Here's how the part is built. I have some questions about the finished solid (model axes, mm). A direction names the side the tool comes from. Give positions to 0.01 mm unless a question says otherwise; leave off trailing zeros. Order: outer loops, then holes, each group sorted by start corner. A loop starts at its lowest first (then second) coordinate and runs counter-clockwise, first axis right, second up.
Autodesk Inventor part; units mm, degrees
ref_plane "YZ Plane" through (0, 0, 0) normal (1, 0, 0) x (0, 1, 0)
ref_plane "XZ Plane" through (0, 0, 0) normal (0, 1, 0) x (-1, 0, 0)
ref_plane "XY Plane" through (0, 0, 0) normal (0, 0, 1) x (1, 0, 0)
sketch "Sketch1" plane through (0, 0, 0) normal (1, 0, 0) x (0, 1, 0)
  line L0 (0, 0) -> (0, 8)
  line L1 (0, 8) -> (2.5, 8)
  circle A0 centre (2.5, 8) radius 1.05
  circle A1 centre (2.5, 8) radius 1.9
  dimension "d1" = 8
  dimension "d2" = 2.5
  dimension "d3" = 2.1
  dimension "d7" = 3.8
sketch "Sketch4" plane through (0, 0, 0) normal (1, 0, 0) x (0, 1, 0)
  line L0 (0, 0) -> (0, 3.5)
  line L1 (0, 3.5) -> (0, 12.5)
  line L2 (0, 12.5) -> (2.5, 12.5)
  line L3 (2.5, 12.5) -> (5.5, 12.5)
  line L4 (5.5, 12.5) -> (5.5, 9.5)
  line L5 (2.5, 12.5) -> (5.5, 9.5)
  line L6 (0, 0) -> (5.5, 0)
  line L7 (5.5, 0) -> (5.5, 9.5)
  dimension "d32" = 3.5
  dimension "d33" = 9
  dimension "d35" = 2.5
  dimension "d37" = 3
  dimension "d38" = 3
extrude "Extrusion3" add sketch "Sketch4" along normal blind 3 contours L0 L1 L2 L5 L7 L6
sketch "Sketch9" plane through (3, 0, 0) normal (1, 0, 0) x (0, 0, -1)
  line L0 (0, 0) -> (-3.5, 0)
  line L1 (-12.5, 0) -> (0, 0)
  line L2 (-3.5, 0) -> (-4.5, 0)
  line L3 (-3.5, 0) -> (-3.5, 2.5)
  line L4 (-3.5, 2.5) -> (-4.5, 2.5)
  line L5 (-4.5, 2.5) -> (-4.5, 0)
  line L6 (-4.5, 0) -> (-11.5, 0)
  line L7 (-11.5, 2.5) -> (-12.5, 2.5)
  line L8 (-11.5, 2.5) -> (-11.5, 0)
  line L9 (-12.5, 2.5) -> (-12.5, 0)
  line L10 (-12.5, 0) -> (-11.5, 0)
  dimension "d70" = 3.5
  dimension "d71" = 1
  dimension "d72" = 1
  dimension "d73" = 7
  dimension "d74" = 2.5
extrude "Extrusion4" add sketch "Sketch9" along normal blind 2 contours L9 L7 L8 L1
sketch "Sketch10" plane through (0, 0, 12.5) normal (0, 0, 1) x (1, 0, 0)
  line L0 (3, 0) -> (3, 5.5)
  line L1 (3, 0) -> (5, 0)
  line L2 (3, 0) -> (3, 2.5)
  line L3 (3, 2.5) -> (5, 2.5)
  line L4 (5, 2.5) -> (5, 0)
  line L5 (3, 2.5) -> (5, 0)
  point P0 (0, 0)
  dimension "d110" = 2
  dimension "d111" = 2.5
extrude "Extrusion9" cut sketch "Sketch10" against normal blind 1 contours L3 L4 L5
hole "Hole5" at (0, 2.5, 8) direction (1, 0, 0) diameter 3.8 depth 1.2
hole "Hole6" at (0, 2.5, 8) direction (1, 0, 0) diameter 2.1 end through all
mirror "Mirror3" about plane through (0, 0, 0) normal (0, 0, 1) of "Extrusion3", "Extrusion4", "Extrusion9", "Hole5", "Hole6"
equation "\"d38\" = d37"
equation "\"d90\" = d7"
equation "\"d97\" = d3"
properties part number "holes"
Q1. If we section it at D-D on x = 2.75: List the corners of the cut face in (y, z) for me, plus the area to 3 significant figures.
Filled sheet:
outline: (0, -12.5) - (2.5, -12.5) - (5.5, -9.5) - (5.5, 9.5) - (2.5, 12.5) - (0, 12.5) - close; hole circle Ø2.1 at (2.5, -8); hole circle Ø2.1 at (2.5, 8)
area: 122 mm2
Q2. For faces 1 (the face through (1.2, 2.5, -6.8)), 2 (the face through (4, 1, -11.5)), 3 (the face through (0, 3, 0)), which set-ups out of +Z, -Z, +X, -X, +Y, -Y let a thin tool reach every point of the face, with its end or its side?
Filled sheet:
face 1: -X
face 2: +X, +Y, -Y
face 3: +Z, -Z, -X, +Y, -Y
Q3. I'm going to push flat-ended pins straight in: P1, Ø3, axis at y = 2.5, z = 8, coming from the -X side; P2, Ø2.5, axis at y = 2.5, z = -8, coming from the +X side. Where does each tip first touch, or does it pass through?
Filled sheet:
P1: stops at x = 1.2
P2: stops at x = 3
Q4. I need wall thicknesses on L1, parallel to Z at x = 3.6, y = 0.65; L2, parallel to Y at x = 0.8, z = 8; L3, parallel to X at y = 2.55, z = -5.5. Which ranges of each line are inside material? Lowest first, please.
Filled sheet:
L1: z = -12.5 to -11.5, 11.5 to 12.5
L2: y = 0 to 0.6, 4.4 to 5.5
L3: x = 0 to 3
Q5. Thinking about a two-plate mould opening in Z: for faces 4 (the face through (2.11, 3.54, -7.86)), 5 (the face through (3.986, 1.268, 12.007)), 6 (the face through (2, 1, 12.5)), 7 (the face through (4, 1, 11.5)), which applies, released by +Z, released by -Z, zero draft, split by the parting line, or undercut?
Filled sheet:
face 4: undercut
face 5: zero draft
face 6: released by +Z
face 7: undercut
Q6. If we section it at A-A on z = -8: List the corners of the cut face in (x, y) for me.
Filled sheet:
outline: (0, 0) - (3, 0) - (3, 1.45) - (1.2, 1.45) - (1.2, 0.6) - (0, 0.6) - close; (0, 4.4) - (1.2, 4.4) - (1.2, 3.55) - (3, 3.55) - (3, 5.5) - (0, 5.5) - close
Q7. If we section it at B-B on y = 3.1: List the corners of the cut face in (x, z) for me, plus the area to 3 significant figures.
Filled sheet:
outline: (0, -11.9) - (3, -11.9) - (3, -8.86) - (1.2, -8.86) - (1.2, -9.8) - (0, -9.8) - close; (0, -6.2) - (1.2, -6.2) - (1.2, -7.14) - (3, -7.14) - (3, 7.14) - (1.2, 7.14) - (1.2, 6.2) - (0, 6.2) - close; (0, 9.8) - (1.2, 9.8) - (1.2, 8.86) - (3, 8.86) - (3, 11.9) - (0, 11.9) - close
area: 56.5 mm2
Q8. If we section it at C-C on x = 4.15: List the corners of the cut face in (y, z) for me.
Filled sheet:
outline: (0, -12.5) - (1.06, -12.5) - (1.06, -11.5) - (0, -11.5) - close; (0, 11.5) - (1.06, 11.5) - (1.06, 12.5) - (0, 12.5) - close
